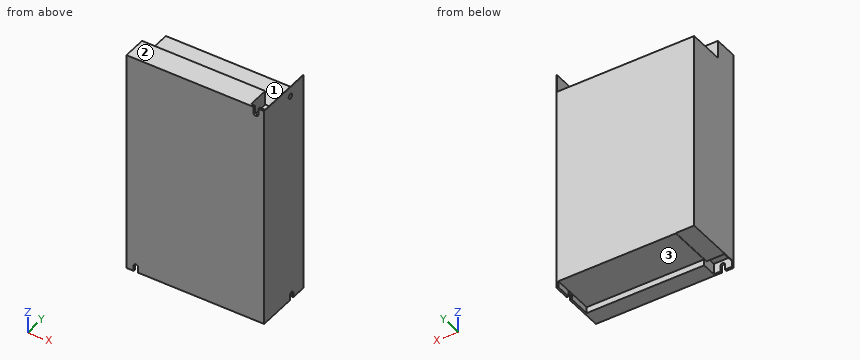
from build123d import *

# Parameters (mm, degrees)
SKETCH1_W           = 97.6884
SKETCH1_H           = 158.75
BOSS_EXTRUDE1_DEPTH = 42
CUT_EXTRUDE1_START  = -97.6884
SKETCH2_W           = 12.7
SKETCH2_H           = 25.4
CUT_EXTRUDE1_DEPTH  = 97.4344
SKETCH3_W           = 10.0203
SKETCH3_H           = 10.1346
CUT_EXTRUDE2_DEPTH  = 15.076
SKETCH4_W           = 13.0175
SKETCH4_H           = 4.6609
CUT_EXTRUDE3_DEPTH  = 40.476
SKETCH5_W           = 12.5095
SKETCH5_H           = 7.62
CUT_EXTRUDE4_DEPTH  = 7.62
SKETCH6_W           = 96.3549
SKETCH6_H           = 4.3815
CUT_EXTRUDE5_DEPTH  = 30.2133
CUT_EXTRUDE6_DEPTH  = 191.743001367
CUT_EXTRUDE7_DEPTH  = 1.3335
SKETCH9_R           = 1.778
CUT_EXTRUDE8_DEPTH  = 0.254
CUT_EXTRUDE9_DEPTH  = 1.524


with BuildPart() as part:
    # Sketch1 → Boss-Extrude1 (new body)
    with BuildSketch(Plane(origin=(0, 0, 0), x_dir=(1, 0, 0), z_dir=(0, 1, 0))):
        with Locations((48.8442, 79.375)):
            Rectangle(SKETCH1_W, SKETCH1_H)
    extrude(amount=BOSS_EXTRUDE1_DEPTH)

    # Sketch2 → Cut-Extrude1 (cut)
    with BuildSketch(Plane(origin=(97.6884, 0, 0), x_dir=(0, 0, -1), z_dir=(1, 0, 0)).offset(CUT_EXTRUDE1_START)):
        with Locations((6.35, 29.3)):
            Rectangle(SKETCH2_W, SKETCH2_H)
    extrude(amount=CUT_EXTRUDE1_DEPTH, mode=Mode.SUBTRACT)

    # Sketch3 → Cut-Extrude2 (cut)
    with BuildSketch(Plane(origin=(0, 16.6, 0), x_dir=(1, 0, 0), z_dir=(0, 1, 0))):
        with Locations((92.42425, 5.0673)):
            Rectangle(SKETCH3_W, SKETCH3_H)
    extrude(amount=-CUT_EXTRUDE2_DEPTH, mode=Mode.SUBTRACT)

    # Sketch4 → Cut-Extrude3 (cut)
    with BuildSketch(Plane(origin=(0, 42, 0), x_dir=(1, 0, 0), z_dir=(0, 1, 0))):
        with Locations((6.50875, 156.41955)):
            Rectangle(SKETCH4_W, SKETCH4_H)
    extrude(amount=-CUT_EXTRUDE3_DEPTH, mode=Mode.SUBTRACT)

    # Sketch5 → Cut-Extrude4 (cut)
    with BuildSketch(Plane(origin=(0, 1.524, 0), x_dir=(1, 0, 0), z_dir=(0, 1, 0))):
        with Locations((6.76275, 154.94)):
            Rectangle(SKETCH5_W, SKETCH5_H)
    extrude(amount=CUT_EXTRUDE4_DEPTH, mode=Mode.SUBTRACT)

    # Sketch6 → Cut-Extrude5 (cut)
    with BuildSketch(Plane(origin=(0, 42, 0), x_dir=(1, 0, 0), z_dir=(0, 1, 0))):
        with Locations((48.17745, 156.55925)):
            Rectangle(SKETCH6_W, SKETCH6_H)
    extrude(amount=-CUT_EXTRUDE5_DEPTH, mode=Mode.SUBTRACT)

    # Sketch7 → Cut-Extrude6 (cut, through all)
    with BuildSketch(Plane(origin=(0, 1.524, 0), x_dir=(1, 0, 0), z_dir=(0, 1, 0))):
        with BuildLine():
            Line((5.08, 158.75), (5.08, 154.813))
            ThreePointArc((5.08, 154.813), (6.6675, 153.2255), (8.255, 154.813))
            Line((8.255, 154.813), (8.255, 158.75))
            Line((8.255, 158.75), (5.08, 158.75))
        make_face()
    extrude(amount=-CUT_EXTRUDE6_DEPTH, mode=Mode.SUBTRACT)

    # Sketch8 → Cut-Extrude7 (cut)
    with BuildSketch(Plane(origin=(97.6884, 0, 0), x_dir=(0, 0, -1), z_dir=(1, 0, 0))):
        with BuildLine():
            Line((158.75, 31.1288), (155.2829, 31.1288))
            ThreePointArc((155.2829, 31.1288), (153.47315, 29.31905), (155.2829, 27.5093))
            Line((155.2829, 27.5093), (158.75, 27.5093))
            Line((158.75, 27.5093), (158.75, 31.1288))
        make_face()
    extrude(amount=-CUT_EXTRUDE7_DEPTH, mode=Mode.SUBTRACT)

    # Sketch9 → Cut-Extrude8 (cut)
    with BuildSketch(Plane(origin=(97.6884, 0, 0), x_dir=(0, 0, -1), z_dir=(1, 0, 0))):
        with Locations((6.858, 27.9665)):
            Circle(SKETCH9_R)
    extrude(amount=-CUT_EXTRUDE8_DEPTH, mode=Mode.SUBTRACT)

    # Sketch10 → Cut-Extrude9 (cut)
    with BuildSketch(Plane.XZ):
        with BuildLine():
            Line((93.5482, 0), (90.1446, 0))
            Line((90.1446, 0), (90.1446, -4.445))
            ThreePointArc((90.1446, -4.445), (91.8464, -6.1468), (93.5482, -4.445))
            Line((93.5482, -4.445), (93.5482, 0))
        make_face()
    extrude(amount=-CUT_EXTRUDE9_DEPTH, mode=Mode.SUBTRACT)


solid = part.part
Check sheet for the modelled part. Datum: model origin and axes. Units: mm. Face numbers are marked on the shaded views. A direction names the side the tool comes from. Round coordinates to 2 decimals unless told otherwise and drop trailing zeros. Loops run counter-clockwise (first coordinate to the right, second up) from the corner with the lowest first, then second, coordinate; pieces in that order, holes last. Notation, with made-up numbers: M 77.25,86 L 85.25,86 A27 ccw 85.25,112 Z; hole C 8,79 d3. An arc over 180 degrees is marked long. One line per question, with ' | ' between items. Start each with the question number.
Item 1: Section check B-B (y = 13.5). Record the boundary of the cut face in (x, z), and give its area (3 significant figures).
Item 2: Section check C-C (x = 62.5). Record the boundary of the cut face in (y, z), and give its area (3 significant figures).
Item 3: Section check A-A (x = 10). Record the boundary of the cut face in (y, z).
Item 4: Set-up check for the marked faces 1, 2 and 3: record each of +Z, -Z, +X, -X, +Y, -Y from which the full face is reachable in a straight line by a thin tool's end or side.
Item 5: Scan lines: probe 1 along Z at (x, y) = (54, 37.5); probe 2 along Z at (x, y) = (7.5, 20.5). Record each from-to range of solid material in increasing order.
Item 6: Gauge pin test, flat ends, axial feed: pin 1 Ø1.3 at (y, z) = (23, -156) entering from -X; pin 2 Ø8 at (x, z) = (90, -6.5) entering from +Y; pin 3 Ø10.5 at (x, y) = (4.5, 30) entering from -Z. Record the tip position at first contact, or that the pin passes through.
Item 7: Section check D-D (y = 39). Record the boundary of the cut face in (x, z).
Worked out:
1) outline: M 0,-154.09 L 13.02,-154.09 L 13.02,-154.37 L 96.35,-154.37 L 96.35,-158.75 L 97.69,-158.75 L 97.69,0 L 97.43,0 L 97.43,-10.13 L 87.41,-10.13 L 87.41,0 L 0,0 Z | area: 15,000 mm^2
2) outline: M 0,-158.75 L 11.79,-158.75 L 11.79,-154.37 L 42,-154.37 L 42,-12.7 L 16.6,-12.7 L 16.6,0 L 0,0 Z | area: 6,210 mm^2
3) outline: M 0,-158.75 L 1.52,-158.75 L 1.52,-151.13 L 9.14,-151.13 L 9.14,-154.09 L 42,-154.09 L 42,-12.7 L 16.6,-12.7 L 16.6,0 L 0,0 Z
4) face 1: +Z, -X, +Y | face 2: +Z, +X, -X, +Y, -Y | face 3: -Z, -X, +Y
5) probe 1: -154.37 to -12.7 | probe 2: -154.09 to -12.7
6) pin 1: x = 96.35 | pin 2: y = 16.6 | pin 3: z = -154.09
7) outline: M 0,-154.09 L 13.02,-154.09 L 13.02,-154.37 L 96.35,-154.37 L 96.35,-158.75 L 97.69,-158.75 L 97.69,0 L 97.43,0 L 97.43,-12.7 L 0,-12.7 Z
